from build123d import *

# Parameters (mm, degrees)
EXTRUDE_1_DEPTH             = 90
SKETCH_2_W                  = 90
SKETCH_2_H                  = 17.75
EXTRUDE_2_DEPTH             = 8.2
SKETCH_3_W                  = 90
SKETCH_3_H                  = 50.95
EXTRUDE_3_DEPTH             = 8.2
SKETCH_4_W                  = 3.95
SKETCH_4_H                  = 29.5
CUT_EXTRUDE_1_DEPTH         = 96.44153315
SKETCH_5_W                  = 3.95
SKETCH_5_H                  = 6.2
CUT_EXTRUDE_2_DEPTH         = 96.44153315
SKETCH_6_W                  = 2.25
SKETCH_6_H                  = 3.95
CUT_EXTRUDE_3_DEPTH         = 96.44153315
SKETCH_7_W                  = 4.5
SKETCH_7_H                  = 3.95
CUT_EXTRUDE_4_DEPTH         = 96.44153315
SKETCH_8_W                  = 2.25
SKETCH_8_H                  = 3.95
CUT_EXTRUDE_5_DEPTH         = 96.44153315
SKETCH_9_W                  = 3.95
SKETCH_9_H                  = 2.25
CUT_EXTRUDE_6_DEPTH         = 96.44153315
SKETCH_10_W                 = 20.2
SKETCH_10_H                 = 45.2
CUT_EXTRUDE_7_DEPTH         = 86
HOLE_WIZARD_2_5_2_5_1_D     = 2.5
HOLE_WIZARD_4_5_4_5_1_D     = 4.5
HOLE_WIZARD_8_3_8_3_1_D     = 8.3
HOLE_WIZARD_8_3_8_3_1_DEPTH = 3.2
FILLET_1_R                  = 2
FILLET_2_R                  = 2
EXTRUDE_START               = -90
SKETCH_17_R                 = 1.25
EXTRUDE_4_DEPTH             = 90
CUT_EXTRUDE_START           = -100
SKETCH_18_R                 = 4.15
CUT_EXTRUDE_8_DEPTH         = 100
CUT_EXTRUDE_11_DEPTH        = 108
CUT_EXTRUDE_12_DEPTH        = 108
SKETCH_21_W                 = 90
SKETCH_21_H                 = 47
EXTRUDE_5_DEPTH             = 2


with BuildPart() as part:
    # Эскиз1 → Бобышка-Вытянуть1 (new body)
    with BuildSketch(Plane(origin=(90, 0, 0), x_dir=(0, 0, -1), z_dir=(1, 0, 0))):
        with BuildLine():
            Line((6.75, -24.093761792), (6.75, 19.25))
            Line((6.75, 19.25), (-11.593761792, 19.25))
            ThreePointArc((-11.593761792, 19.25), (-15.325, 18), (-11.593761792, 16.75))
            Line((-11.593761792, 16.75), (-11, 16.75))
            Line((-11, 16.75), (-11, -16.75))
            Line((-11, -16.75), (-11.593761792, -16.75))
            ThreePointArc((-11.593761792, -16.75), (-15.325, -18), (-11.593761792, -19.25))
            Line((-11.593761792, -19.25), (-11, -19.25))
            Line((-11, -19.25), (-11, -23.5))
            Line((-11, -23.5), (-6.75, -23.5))
            Line((-6.75, -23.5), (-6.75, -24.093761792))
            ThreePointArc((-6.75, -24.093761792), (-5.5, -27.825), (-4.25, -24.093761792))
            Line((-4.25, -24.093761792), (-4.25, -23.5))
            Line((-4.25, -23.5), (4.25, -23.5))
            Line((4.25, -23.5), (4.25, -24.093761792))
            ThreePointArc((4.25, -24.093761792), (5.5, -27.825), (6.75, -24.093761792))
        make_face()
    extrude(amount=-EXTRUDE_1_DEPTH)

    # Эскиз2 → Бобышка-Вытянуть2 (add)
    with BuildSketch(Plane(origin=(0, 19.25, 0), x_dir=(-1, 0, 0), z_dir=(0, 1, 0))):
        with Locations((-45, 2.125)):
            Rectangle(SKETCH_2_W, SKETCH_2_H)
    extrude(amount=EXTRUDE_2_DEPTH)

    # Эскиз3 → Бобышка-Вытянуть3 (add)
    with BuildSketch(Plane(origin=(0, 0, -6.75), x_dir=(-1, 0, 0), z_dir=(0, 0, -1))):
        with Locations((-45, 1.975)):
            Rectangle(SKETCH_3_W, SKETCH_3_H)
    extrude(amount=EXTRUDE_3_DEPTH)

    # Эскиз4 → Вырез-Вытянуть1 (cut, through all)
    with BuildSketch(Plane.ZY):
        with Locations((-12.975, 0)):
            Rectangle(SKETCH_4_W, SKETCH_4_H)
    extrude(amount=-CUT_EXTRUDE_1_DEPTH, mode=Mode.SUBTRACT)

    # Эскиз5 → Вырез-Вытянуть2 (cut, through all)
    with BuildSketch(Plane.ZY):
        with Locations((-12.975, 24.35)):
            Rectangle(SKETCH_5_W, SKETCH_5_H)
    extrude(amount=-CUT_EXTRUDE_2_DEPTH, mode=Mode.SUBTRACT)

    # Эскиз6 → Вырез-Вытянуть3 (cut, through all)
    with BuildSketch(Plane.ZY):
        with Locations((-9.875, 25.475)):
            Rectangle(SKETCH_6_W, SKETCH_6_H)
    extrude(amount=-CUT_EXTRUDE_3_DEPTH, mode=Mode.SUBTRACT)

    # Эскиз7 → Вырез-Вытянуть4 (cut, through all)
    with BuildSketch(Plane.ZY):
        with Locations((0, 25.475)):
            Rectangle(SKETCH_7_W, SKETCH_7_H)
    extrude(amount=-CUT_EXTRUDE_4_DEPTH, mode=Mode.SUBTRACT)

    # Эскиз8 → Вырез-Вытянуть5 (cut, through all)
    with BuildSketch(Plane.ZY):
        with Locations((9.875, 25.475)):
            Rectangle(SKETCH_8_W, SKETCH_8_H)
    extrude(amount=-CUT_EXTRUDE_5_DEPTH, mode=Mode.SUBTRACT)

    # Эскиз9 → Вырез-Вытянуть6 (cut, through all)
    with BuildSketch(Plane.ZY):
        with Locations((-12.975, -22.375)):
            Rectangle(SKETCH_9_W, SKETCH_9_H)
    extrude(amount=-CUT_EXTRUDE_6_DEPTH, mode=Mode.SUBTRACT)

    # Эскиз10 → Вырез-Вытянуть7 (cut)
    with BuildSketch(Plane(origin=(90, 0, 0), x_dir=(0, 0, -1), z_dir=(1, 0, 0))):
        Rectangle(SKETCH_10_W, SKETCH_10_H)
    extrude(amount=-CUT_EXTRUDE_7_DEPTH, mode=Mode.SUBTRACT)

    # Диаметр отверстия Ø2.5 (2.5)1 (through all)
    with Locations(Plane(origin=(90, 0, 0), x_dir=(0, 0, -1), z_dir=(1, 0, 0))):
        with Locations((5.5, -25.75), (-13.25, -18), (-5.5, -25.75), (-13.25, 18)):
            Hole(HOLE_WIZARD_2_5_2_5_1_D / 2)

    # Диаметр отверстия Ø4.5 (4.5)1 (through all)
    with Locations(Plane.ZY):
        with Locations((-13.25, -18), (-13.25, 18), (-5.5, 25.75), (5.5, 25.75)):
            Hole(HOLE_WIZARD_4_5_4_5_1_D / 2)

    # Диаметр отверстия Ø8.3 (8.3)1
    with Locations(Plane.ZY):
        with Locations((0, 0)):
            Hole(HOLE_WIZARD_8_3_8_3_1_D / 2, depth=HOLE_WIZARD_8_3_8_3_1_DEPTH)

    # Скругление1
    fillet_1_edges = [part.edges().sort_by_distance(p)[0] for p in [
        (45, 23.5, 8.75),
    ]]
    fillet(fillet_1_edges, radius=FILLET_1_R)

    # Скругление2
    fillet_2_edges = [part.edges().sort_by_distance(p)[0] for p in [
        (45, 23.5, -8.75),
        (45, 23.5, 2.25),
        (45, 23.5, -2.25),
        (45, -21.25, -11),
        (4, 0, -10.1),
        (4, -22.6, 0),
        (4, 0, 10.1),
        (4, 22.6, 0),
        (45, 14.75, -11),
        (45, -14.75, -11),
        (45, 21.25, -11),
    ]]
    fillet(fillet_2_edges, radius=FILLET_2_R)

    # Эскиз17 → Бобышка-Вытянуть4 (add)
    with BuildSketch(Plane(origin=(90, 0, 0), x_dir=(0, 0, -1), z_dir=(1, 0, 0)).offset(EXTRUDE_START)):
        with Locations((5.5, -25.75)):
            Circle(SKETCH_17_R)
        with Locations((-5.5, -25.75)):
            Circle(SKETCH_17_R)
        with Locations((-13.25, -18)):
            Circle(SKETCH_17_R)
        with Locations((-13.25, 18)):
            Circle(SKETCH_17_R)
    extrude(amount=EXTRUDE_4_DEPTH)

    # Эскиз18 → Вырез-Вытянуть8 (cut)
    with BuildSketch(Plane.ZY.offset(CUT_EXTRUDE_START)):
        Circle(SKETCH_18_R)
    extrude(amount=CUT_EXTRUDE_8_DEPTH, mode=Mode.SUBTRACT)

    # Эскиз19 → Вырез-Вытянуть11 (cut)
    with BuildSketch(Plane(origin=(90, 0, 0), x_dir=(0, 0, -1), z_dir=(1, 0, 0))):
        Polygon((-10.1, -22.6), (-10.1, 22.6), (-10.1, 31.781046402), (18.117629079, 31.781046402), (18.667008159, -30.769686003), (-10.1, -30.769686003), align=None)
    extrude(amount=-CUT_EXTRUDE_11_DEPTH, mode=Mode.SUBTRACT)

    # Эскиз20 → Вырез-Вытянуть12 (cut)
    with BuildSketch(Plane(origin=(90, 0, 0), x_dir=(0, 0, -1), z_dir=(1, 0, 0))):
        with BuildLine():
            Line((-10.75, 23.5), (-10.1, 23.5))
            Line((-10.1, 23.5), (-10.1, 23.608571968))
            ThreePointArc((-10.1, 23.608571968), (-10.420497393, 23.52732972), (-10.75, 23.5))
        make_face()
    extrude(amount=-CUT_EXTRUDE_12_DEPTH, mode=Mode.SUBTRACT)

    # Эскиз21 → Бобышка-Вытянуть5 (add)
    with BuildSketch(Plane(origin=(0, 0, 10.1), x_dir=(-1, 0, 0), z_dir=(0, 0, -1))):
        with Locations((-45, 0)):
            Rectangle(SKETCH_21_W, SKETCH_21_H)
    extrude(amount=EXTRUDE_5_DEPTH)


solid = part.part
Could you check a few things on this model? Use its own coordinates, in mm. A direction names the side the tool comes from. Give positions to 0.01 mm unless a question says otherwise; leave off trailing zeros. Order: outer loops, then holes, each group sorted by start corner. A loop starts at its lowest first (then second) coordinate and runs counter-clockwise, first axis right, second up. Notation, with made-up numbers: (-6.5, 13) - (11.5, 13) arc R18 ccw to (11.5, 29) - close; hole circle Ø8 at (47.5, -9). An arc over 180 degrees is marked (long way). One line per question, with ' | ' between items. Start each with the question number.
Item 1: I want a section at C-C on y = 5.5. Write out the boundary of the cut face in (x, z), then the cut area to 3 significant figures.
Item 2: I'm going to push flat-ended pins straight in: pin 1 Ø10 at (x, y) = (25.5, -10) entering from +Z; pin 2 Ø0.7 at (x, z) = (31.5, 11.5) entering from -Y; pin 3 Ø2 at (x, z) = (49, 13) entering from -Y (3 decimals). Where does each tip first touch, or does it pass through?
Item 3: I want a section at B-B on x = 83. Write out the boundary of the cut face in (y, z) (3 decimals).
Item 4: I need wall thicknesses on probe 1 along Z at (x, y) = (63, 5); probe 2 along Y at (x, z) = (25.5, 13.5); probe 3 along Y at (x, z) = (80, 14). Which ranges of each line are inside material? Lowest first, please. Write a range as [from, to].
Item 5: For faces 1 (the flat face through (46, 21, 11)), 2 (the cylindrical face through (45.63, 18.072, 15.324)), which set-ups out of +Z, -Z, +X, -X, +Y, -Y let a thin tool reach every point of the face, with its end or its side?
Item 6: Thinking about a two-plate mould opening in Y: for faces 3 (the flat face through (46, 23.5, 10)), 4 (the flat face through (46, -21, 11)), 5 (the cylindrical face through (45.63, -17.928, 15.324)), 6 (the flat face through (46, 0, 11)), which applies, pulls with the +Y half, pulls with the -Y half, needs draft (parallel to the pull), parting line crosses it, or undercut?
Item 7: I want a section at A-A on z = 13.25. Write out the boundary of the cut face in (x, y) (3 decimals), then the cut area to 3 significant figures.
Verdict:
1) outline: (0, 8.1) - (90, 8.1) - (90, 11) - (0, 11) - close | area: 261 mm^2
2) pin 1: z = 11 | pin 2: y = -19.53 | pin 3: y = -20.075
3) outline: (-23.5, 8.1) - (23.5, 8.1) - (23.5, 11) - (19.25, 11) - (19.25, 11.594) arc R2.075 ccw (long way) to (16.75, 11.594) - (16.75, 11) - (-16.75, 11) - (-16.75, 11.594) arc R2.075 ccw (long way) to (-19.25, 11.594) - (-19.25, 11) - (-23.5, 11) - close
4) probe 1: [8.1, 11] | probe 2: [-20.06, -15.94], [15.94, 20.06] | probe 3: [-19.93, -16.07], [16.07, 19.93]
5) face 1: +X, -X, +Y | face 2: +X, -X
6) face 3: pulls with the +Y half | face 4: needs draft | face 5: undercut | face 6: undercut
7) outline: (0, -20.075) - (90, -20.075) - (90, -15.925) - (0, -15.925) - close; (0, 15.925) - (90, 15.925) - (90, 20.075) - (0, 20.075) - close | area: 747 mm^2
